```python
from build123d import *

# Parameters (mm, degrees)
IZIM1_W                     = 77.58
IZIM1_H                     = 160.7
Y_KSEKLIK_EKSTR_ZYON1_DEPTH = 7.85
RADYUS1_R                   = 10
Y_KSEKLIK_EKSTR_ZYON2_DEPTH = 2
Y_KSEKLIK_EKSTR_ZYON3_DEPTH = 1
RADYUS3_R                   = 0.8


with BuildPart() as part:
    # Çizim1 → Yükseklik-Ekstrüzyon1 (new body)
    with BuildSketch(Plane.XY):
        with Locations((15.94448574, -50.114448669)):
            Rectangle(IZIM1_W, IZIM1_H)
    extrude(amount=Y_KSEKLIK_EKSTR_ZYON1_DEPTH)

    # Radyus1
    radyus1_edges = [part.edges().sort_by_distance(p)[0] for p in [
        (-22.84551426, 30.235551331, 3.925),
        (54.73448574, 30.235551331, 3.925),
        (54.73448574, -130.464448669, 3.925),
        (-22.84551426, -130.464448669, 3.925),
    ]]
    fillet(radyus1_edges, radius=RADYUS1_R)

    # Çizim3 → Yükseklik-Ekstrüzyon2 (add)
    with BuildSketch(Plane(origin=(0, 0, 0), x_dir=(-1, 0, 0), z_dir=(0, 0, -1))):
        with BuildLine():
            Line((-42.73448574, 28.235551331), (-22.73448574, 28.235551331))
            ThreePointArc((-22.73448574, 28.235551331), (-15.663417928, 25.306619143), (-12.73448574, 18.235551331))
            Line((-12.73448574, 18.235551331), (-12.73448574, -1.764448669))
            ThreePointArc((-12.73448574, -1.764448669), (-15.663417928, -8.835516481), (-22.73448574, -11.764448669))
            Line((-22.73448574, -11.764448669), (-42.73448574, -11.764448669))
            ThreePointArc((-42.73448574, -11.764448669), (-49.805553552, -8.835516481), (-52.73448574, -1.764448669))
            Line((-52.73448574, -1.764448669), (-52.73448574, 18.235551331))
            ThreePointArc((-52.73448574, 18.235551331), (-49.805553552, 25.306619143), (-42.73448574, 28.235551331))
        make_face()
    extrude(amount=Y_KSEKLIK_EKSTR_ZYON2_DEPTH)

    # Çizim7 → Yükseklik-Ekstrüzyon3 (add)
    with BuildSketch(Plane(origin=(0, 0, -2), x_dir=(-1, 0, 0), z_dir=(0, 0, -1))):
        with BuildLine():
            Line((-42.73448574, 27.235551331), (-22.73448574, 27.235551331))
            ThreePointArc((-22.73448574, 27.235551331), (-16.370524709, 24.599512361), (-13.73448574, 18.235551331))
            Line((-13.73448574, 18.235551331), (-13.73448574, -1.764448669))
            ThreePointArc((-13.73448574, -1.764448669), (-16.370524709, -8.1284097), (-22.73448574, -10.764448669))
            Line((-22.73448574, -10.764448669), (-42.73448574, -10.764448669))
            ThreePointArc((-42.73448574, -10.764448669), (-49.098446771, -8.1284097), (-51.73448574, -1.764448669))
            Line((-51.73448574, -1.764448669), (-51.73448574, 18.235551331))
            ThreePointArc((-51.73448574, 18.235551331), (-49.098446771, 24.599512361), (-42.73448574, 27.235551331))
        make_face()
    extrude(amount=Y_KSEKLIK_EKSTR_ZYON3_DEPTH)

    # Radyus3
    radyus3_edges = [part.edges().sort_by_distance(p)[0] for p in [
        (49.805553552, 25.306619143, -2),
        (52.73448574, 8.235551331, -2),
        (49.805553552, -8.835516481, -2),
        (32.73448574, -11.764448669, -2),
        (15.663417928, -8.835516481, -2),
        (12.73448574, 8.235551331, -2),
        (15.663417928, 25.306619143, -2),
        (32.73448574, 28.235551331, -2),
    ]]
    fillet(radyus3_edges, radius=RADYUS3_R)


solid = part.part
```
Input: part model. Units: mm. Frame: model coordinates. A direction names the side the tool comes from. Give positions to 0.01 mm unless a question says otherwise; leave off trailing zeros. Order: outer loops, then holes, each group sorted by start corner. A loop starts at its lowest first (then second) coordinate and runs counter-clockwise, first axis right, second up. Notation, with made-up numbers: M 23,17.5 L 65,17.5 A30 cw 65,48.5 Z; hole C 49.25,45.25 d10. An arc over 180 degrees is marked long. One line per question, with ' | ' between items. Start each with the question number.
1. First-contact query: pin 1 Ø12 at (x, y) = (9, -32.5) entering from -Z; pin 2 Ø0.6 at (y, z) = (5.5, -0.5) entering from -X; pin 3 Ø2 at (y, z) = (-109, -1.5) entering from +X; pin 4 Ø0.6 at (x, z) = (31.5, -0.5) entering from +Y. Flat tips, straight axial feed; report the tip coordinate or a pass-through.
2. Material intervals for probe 1 along Z at (x, y) = (26, -43.5); probe 2 along Y at (x, z) = (-15, 4.5), sorted ascending. Write a range as [from, to].
3. Access query for faces 1 (the face through (49.028, -8.198, -2.493)), 2 (the face through (16.44, 24.67, -2.49)), 3 (the face through (16.301, -8.058, -2.493)). Directions: +Z, -Z, +X, -X, +Y, -Y. A direction counts if a zero-diameter tool reaches every point of the face in a straight line with its end or side. Return the directions, or none.
4. Section query B-B (x = 30.5). Return the cut outline in (y, z).
5. Section query A-A (y = 16.5). Return the cut outline in (x, z).
6. Section query C-C (y = -15.5). Return the cut outline in (x, z).
7. Section query D-D (x = -2). Return the cut outline in (y, z).
Here are the results:
1) pin 1: z = 0 | pin 2: x = 12.73 | pin 3: through | pin 4: y = 28.24
2) probe 1: [0, 7.85] | probe 2: [-130.23, 30]
3) face 1: -Z, +X, -Y | face 2: -Z, -X, +Y | face 3: -Z, -X, -Y
4) outline: M -130.46,0 L -11.76,0 L -11.76,-1.2 A0.8 ccw -10.96,-2 L -10.76,-2 L -10.76,-3 L 27.24,-3 L 27.24,-2 L 27.44,-2 A0.8 ccw 28.24,-1.2 L 28.24,0 L 30.24,0 L 30.24,7.85 L -130.46,7.85 Z
5) outline: M -22.85,0 L 12.73,0 L 12.73,-1.2 A0.8 ccw 13.53,-2 L 13.73,-2 L 13.73,-3 L 51.73,-3 L 51.73,-2 L 51.93,-2 A0.8 ccw 52.73,-1.2 L 52.73,0 L 54.73,0 L 54.73,7.85 L -22.85,7.85 Z
6) outline: M -22.85,0 L 54.73,0 L 54.73,7.85 L -22.85,7.85 Z
7) outline: M -130.46,0 L 30.24,0 L 30.24,7.85 L -130.46,7.85 Z
